from build123d import *

# Parameters (mm, degrees)
EXTRUDE_1_DEPTH     = 2.5
SKETCH_2_R          = 1.6
CUT_EXTRUDE_1_DEPTH = 123.090022194
SKETCH_3_R          = 3
CUT_EXTRUDE_2_DEPTH = 1


with BuildPart() as part:
    # 草图1 → 凸台-拉伸1 (new body)
    with BuildSketch(Plane(origin=(0, 0, 0), x_dir=(1, 0, 0), z_dir=(0, 1, 0))):
        with BuildLine():
            Line((26.135435749, 0.2), (100.135435749, 0.2))
            ThreePointArc((100.135435749, 0.2), (103.529548299, 1.60588745), (104.935435749, 5))
            Line((104.935435749, 5), (104.935435749, 17.5))
            ThreePointArc((104.935435749, 17.5), (105.87269405, 19.7627417), (108.135435749, 20.7))
            Line((108.135435749, 20.7), (111.135435749, 20.7))
            ThreePointArc((111.135435749, 20.7), (113.115334737, 21.520101013), (113.935435749, 23.5))
            Line((113.935435749, 23.5), (113.935435749, 26.5))
            ThreePointArc((113.935435749, 26.5), (113.115334737, 28.479898987), (111.135435749, 29.3))
            Line((111.135435749, 29.3), (108.135435749, 29.3))
            ThreePointArc((108.135435749, 29.3), (105.87269405, 30.2372583), (104.935435749, 32.5))
            Line((104.935435749, 32.5), (104.935435749, 39))
            ThreePointArc((104.935435749, 39), (103.529548299, 42.39411255), (100.135435749, 43.8))
            Line((100.135435749, 43.8), (26.135435749, 43.8))
            ThreePointArc((26.135435749, 43.8), (22.7413232, 42.39411255), (21.335435749, 39))
            Line((21.335435749, 39), (21.335435749, 32.5))
            ThreePointArc((21.335435749, 32.5), (20.398177449, 30.2372583), (18.135435749, 29.3))
            Line((18.135435749, 29.3), (15.135435749, 29.3))
            ThreePointArc((15.135435749, 29.3), (13.155536762, 28.479898987), (12.335435749, 26.5))
            Line((12.335435749, 26.5), (12.335435749, 23.5))
            ThreePointArc((12.335435749, 23.5), (13.155536762, 21.520101013), (15.135435749, 20.7))
            Line((15.135435749, 20.7), (18.135435749, 20.7))
            ThreePointArc((18.135435749, 20.7), (20.398177449, 19.7627417), (21.335435749, 17.5))
            Line((21.335435749, 17.5), (21.335435749, 5))
            ThreePointArc((21.335435749, 5), (22.7413232, 1.60588745), (26.135435749, 0.2))
        make_face()
    extrude(amount=EXTRUDE_1_DEPTH)

    # 草图2 → 切除-拉伸1 (cut, through all)
    with BuildSketch(Plane(origin=(0, 2.5, 0), x_dir=(1, 0, 0), z_dir=(0, 1, 0))):
        with Locations(Location((16.635435749, 25, 0), (0, 0, 270))):
            Circle(SKETCH_2_R)
        with Locations(Location((109.635435749, 25, 0), (0, 0, 270))):
            Circle(SKETCH_2_R)
    extrude(amount=-CUT_EXTRUDE_1_DEPTH, mode=Mode.SUBTRACT)

    # 草图3 → 切除-拉伸2 (cut)
    with BuildSketch(Plane(origin=(0, 2.5, 0), x_dir=(1, 0, 0), z_dir=(0, 1, 0))):
        with Locations(Location((16.635435749, 25, 0), (0, 0, 270))):
            Circle(SKETCH_3_R)
        with Locations(Location((109.635435749, 25, 0), (0, 0, 270))):
            Circle(SKETCH_3_R)
    extrude(amount=-CUT_EXTRUDE_2_DEPTH, mode=Mode.SUBTRACT)


solid = part.part
The listing builds one solid part. Answer for the finished solid, in the listing's coordinates (mm). A direction names the side the tool comes from. Give positions to 0.01 mm unless a question says otherwise; leave off trailing zeros. Order: outer loops, then holes, each group sorted by start corner. A loop starts at its lowest first (then second) coordinate and runs counter-clockwise, first axis right, second up. Notation, with made-up numbers: (65.25, 20) - (96.25, 20) arc R17 ccw to (96.25, 45) - close; hole circle Ø7 at (4, 8). An arc over 180 degrees is marked (long way). Use one line per item in the form item = value.
1) Consider probe 1 along X at (y, z) = (0.4, -25); probe 2 along X at (y, z) = (2.35, -25); probe 3 along X at (y, z) = (2.4, -5.5). Determine where each line is inside the solid, lowest interval first. Write a range as [from, to].
Verdict:
probe_1 = [12.34, 15.04], [18.24, 108.04], [111.24, 113.94]
probe_2 = [12.34, 13.64], [19.64, 106.64], [112.64, 113.94]
probe_3 = [21.34, 104.94]
2) The mould has two halves that part along X. Classify faces 4 (the flat face through (62, 2.5, -22)), 5 (the flat face through (15, 1.5, -24)), 6 (the cylindrical face through (103.567, 1.232, -42.357)): released by +X, released by -X, zero draft, split by the parting line, or undercut.
Verdict:
face_4 = zero draft
face_5 = undercut
face_6 = released by +X
3) Find section B-B on y = 2. Determine the outline of the cut face in (x, z), and give its area (3 significant figures).
Verdict:
outline = (12.34, -26.5) arc R2.8 ccw to (15.14, -29.3) - (18.14, -29.3) arc R3.2 cw to (21.34, -32.5) - (21.34, -39) arc R4.8 ccw to (26.14, -43.8) - (100.14, -43.8) arc R4.8 ccw to (104.94, -39) - (104.94, -32.5) arc R3.2 cw to (108.14, -29.3) - (111.14, -29.3) arc R2.8 ccw to (113.94, -26.5) - (113.94, -23.5) arc R2.8 ccw to (111.14, -20.7) - (108.14, -20.7) arc R3.2 cw to (104.94, -17.5) - (104.94, -5) arc R4.8 ccw to (100.14, -0.2) - (26.14, -0.2) arc R4.8 ccw to (21.34, -5) - (21.34, -17.5) arc R3.2 cw to (18.14, -20.7) - (15.14, -20.7) arc R2.8 ccw to (12.34, -23.5) - close; hole circle Ø6 at (16.64, -25); hole circle Ø6 at (109.64, -25)
area = 3,730 mm^2
4) Find section C-C on z = -6. Determine the outline of the cut face in (x, y).
Verdict:
outline = (21.34, 0) - (104.94, 0) - (104.94, 2.5) - (21.34, 2.5) - close
5) Each of these flat-tipped pins is pushed along its axis until it touches: pin 1 (0.8 mm diameter, centred on x = 109.5, y = 1, fed in from -Z); pin 2 (1 mm diameter, centred on x = 103.5, y = 1.5, fed in from +Z); pin 3 (1.2 mm diameter, centred on y = 1.5, z = -13, fed in from +X); pin 4 (1.8 mm diameter, centred on x = 109.5, z = -24.5, fed in from +Y). Where does it stop, or does it pass through?
Verdict:
pin_1 = -29.3
pin_2 = -1.15
pin_3 = 104.94
pin_4 = through
6) Find section A-A on z = -25. Determine the outline of the cut face in (x, y).
Verdict:
outline = (12.34, 0) - (15.04, 0) - (15.04, 1.5) - (13.64, 1.5) - (13.64, 2.5) - (12.34, 2.5) - close; (18.24, 0) - (108.04, 0) - (108.04, 1.5) - (106.64, 1.5) - (106.64, 2.5) - (19.64, 2.5) - (19.64, 1.5) - (18.24, 1.5) - close; (111.24, 0) - (113.94, 0) - (113.94, 2.5) - (112.64, 2.5) - (112.64, 1.5) - (111.24, 1.5) - close
7) For faces 1 (the flat face through (104.935, 1, -36)), 2 (the flat face through (17, 1, -20.7)), 3 (the cylindrical face through (19.61, 2.01, -25.39)), determine the directions among +Z, -Z, +X, -X, +Y, -Y from which every point of the face is accessible in a straight line to the end or side of a thin tool.
Verdict:
face_1 = -Z, +X, +Y, -Y
face_2 = +Z, -X, +Y, -Y
face_3 = +Y
